Geometry: final body of the model. Coordinates: model frame, mm. A direction names the side the tool comes from. Coordinates: 2 decimals unless noted, no trailing zeros. Write each loop counter-clockwise with the first axis right and the second up, starting at its lowest first coordinate (ties: lowest second). Pieces come first, ordered by that corner, then holes. Notation, with made-up numbers: (-6.5, -10.75) - (40.5, -10.75) arc R16 ccw to (40.5, 12.25) - close; hole circle Ø2 at (36.25, -34.75). An arc over 180 degrees is marked (long way). Answer as a JSON object with one key per item and string values. Group by question number.
Item 1: Section C-C on y = 62.15. Return loops of the section in (x, z), and give its area (3 significant figures).
Item 2: Set-up query: faces 1 (the flat face through (30, 70.15, 14)), 2 (the flat face through (54, 6, 25)), 3 (the cylindrical face through (32.494, 27.794, 26.014)). Return all of +Z, -Z, +X, -X, +Y, -Y with unobstructed straight access to the full face (end or side cutting, diameter ignored); none if empty.
Item 3: First-contact query: pin 1 Ø2 at (x, y) = (34, 54) entering from -Z; pin 2 Ø2 at (x, y) = (9, 9.5) entering from +Z; pin 3 Ø3.5 at (x, y) = (8.075, 24) entering from -Z. Flat tips, straight axial feed; report the tip coordinate or a pass-through.
Item 4: Line query: line 1 along Y through (x, z) = (52.15, 24.6); line 2 along Y through (x, z) = (8, 26.2); line 3 along Y through (x, z) = (40.5, 17.75). Output: solid intervals per line, ascending. Write a range as from..to.
Item 5: Mould query, pull axis Y, two halves, no side actions, for faces 4 (the cylindrical face through (11.434, 9.081, 26.014)), 5 (the flat face through (-1.095, -1.148, 13.311)), 6 (the flat face through (59.16, 1.01, 14.37)), 7 (the flat face through (-3, 35, 13)). Classes: pulls with the +Y half, pulls with the -Y half, needs draft (parallel to the pull), parting line crosses it, or undercut.
Item 6: Section A-A on y = 24. State how many separate pieces and enclosed holes the cut face has, and give its area (3 significant figures).
Item 7: Section D-D on z = 2. Return loops of the section in (x, y), and give its area (3 significant figures).
```python
from build123d import *
from OCP.BRepFilletAPI import BRepFilletAPI_MakeChamfer

# Parameters (mm, degrees)
SKIZZE1_W                       = 60.15
SKIZZE1_H                       = 70.15
GRUNDK_RPER_DEPTH               = 24
FASE1_SIZE                      = 2
WANDUNG1_T                      = 3
SKIZZE2_R                       = 4.5
DURCHBRUCH_SERVO_DEPTH          = 101.338651576
SKIZZE4_W                       = 22
SKIZZE4_H                       = 42
SERVOFREISCHNITT_DEPTH          = 1
SCHNITT_LINEAR_AUSTRAGEN2_REACH = 102.339
SKIZZE7_R                       = 2
SKIZZE8_R                       = 3.6
SCHNITT_LINEAR_AUSTRAGEN3_DEPTH = 2
SCHNITT_LINEAR_AUSTRAGEN5_REACH = 102.339
SKIZZE3_R                       = 1.6
FASE2_SIZE                      = 5
FASE2_SIZE2                     = 0.437443318
FASE3_SIZE                      = 1
FASE3_SIZE2                     = 1.100062868


with BuildPart() as part:
    # Skizze1 → Grundkörper (new body)
    with BuildSketch(Plane.XY):
        with Locations((30.075, 35.075)):
            Rectangle(SKIZZE1_W, SKIZZE1_H)
    extrude(amount=GRUNDK_RPER_DEPTH)

    # Fase1
    fase1_edges = [part.edges().sort_by_distance(p)[0] for p in [
        (0, 70.15, 12),
        (60.15, 70.15, 12),
        (60.15, 0, 12),
        (0, 0, 12),
    ]]
    chamfer(fase1_edges, length=FASE1_SIZE)

    # Wandung1
    wandung1_openings = [part.faces().sort_by_distance(p)[0] for p in [
        (30.075, 35.075, 0),
    ]]
    offset(amount=WANDUNG1_T, openings=wandung1_openings, kind=Kind.INTERSECTION)

    # Skizze2 → Durchbruch Servo (cut, through all)
    with BuildSketch(Plane.XY.offset(27)):
        with Locations((30.075, 24)):
            Circle(SKIZZE2_R)
    extrude(amount=-DURCHBRUCH_SERVO_DEPTH, mode=Mode.SUBTRACT)

    # Skizze4 → ServoFreischnitt (cut)
    with BuildSketch(Plane(origin=(0, 0, 24), x_dir=(-1, 0, 0), z_dir=(0, 0, -1))):
        with Locations((-30.075, 35)):
            Rectangle(SKIZZE4_W, SKIZZE4_H)
    extrude(amount=-SERVOFREISCHNITT_DEPTH, mode=Mode.SUBTRACT)

    # Skizze7 → Schnitt-Linear austragen2 (cut, up to next)
    with BuildSketch(Plane.XY.offset(27), mode=Mode.PRIVATE) as schnitt_linear_austragen2_sk1:
        with Locations((8, 62.15)):
            Circle(SKIZZE7_R)
    schnitt_linear_austragen2_tool1 = extrude(schnitt_linear_austragen2_sk1.sketch, amount=-SCHNITT_LINEAR_AUSTRAGEN2_REACH, mode=Mode.PRIVATE) & part.part
    # Skizze7 → Schnitt-Linear austragen2 (cut, up to next)
    with BuildSketch(Plane.XY.offset(27), mode=Mode.PRIVATE) as schnitt_linear_austragen2_sk2:
        with Locations(Location((52.15, 62.15, 0), (0, 0, 180))):
            Circle(SKIZZE7_R)
    schnitt_linear_austragen2_tool2 = extrude(schnitt_linear_austragen2_sk2.sketch, amount=-SCHNITT_LINEAR_AUSTRAGEN2_REACH, mode=Mode.PRIVATE) & part.part
    # Skizze7 → Schnitt-Linear austragen2 (cut, up to next)
    with BuildSketch(Plane.XY.offset(27), mode=Mode.PRIVATE) as schnitt_linear_austragen2_sk3:
        with Locations((52.15, 8)):
            Circle(SKIZZE7_R)
    schnitt_linear_austragen2_tool3 = extrude(schnitt_linear_austragen2_sk3.sketch, amount=-SCHNITT_LINEAR_AUSTRAGEN2_REACH, mode=Mode.PRIVATE) & part.part
    # Skizze7 → Schnitt-Linear austragen2 (cut, up to next)
    with BuildSketch(Plane.XY.offset(27), mode=Mode.PRIVATE) as schnitt_linear_austragen2_sk4:
        with Locations(Location((8, 8, 0), (0, 0, 180))):
            Circle(SKIZZE7_R)
    schnitt_linear_austragen2_tool4 = extrude(schnitt_linear_austragen2_sk4.sketch, amount=-SCHNITT_LINEAR_AUSTRAGEN2_REACH, mode=Mode.PRIVATE) & part.part
    add(schnitt_linear_austragen2_tool1.solids().sort_by_distance((8, 62.15, 27))[0], mode=Mode.SUBTRACT)
    add(schnitt_linear_austragen2_tool2.solids().sort_by_distance((52.15, 62.15, 27))[0], mode=Mode.SUBTRACT)
    add(schnitt_linear_austragen2_tool3.solids().sort_by_distance((52.15, 8, 27))[0], mode=Mode.SUBTRACT)
    add(schnitt_linear_austragen2_tool4.solids().sort_by_distance((8, 8, 27))[0], mode=Mode.SUBTRACT)

    # Skizze8 → Schnitt-Linear austragen3 (cut)
    with BuildSketch(Plane.XY.offset(27)):
        with Locations((8, 62.15)):
            Circle(SKIZZE8_R)
        with Locations((52.15, 62.15)):
            Circle(SKIZZE8_R)
        with Locations((52.15, 8)):
            Circle(SKIZZE8_R)
        with Locations((8, 8)):
            Circle(SKIZZE8_R)
    extrude(amount=-SCHNITT_LINEAR_AUSTRAGEN3_DEPTH, mode=Mode.SUBTRACT)

    # Skizze3 → Schnitt-Linear austragen5 (cut, up to next)
    with BuildSketch(Plane.XY.offset(27), mode=Mode.PRIVATE) as schnitt_linear_austragen5_sk1:
        with Locations((8.075, 24)):
            Circle(SKIZZE3_R)
    schnitt_linear_austragen5_tool1 = extrude(schnitt_linear_austragen5_sk1.sketch, amount=-SCHNITT_LINEAR_AUSTRAGEN5_REACH, mode=Mode.PRIVATE) & part.part
    # Skizze3 → Schnitt-Linear austragen5 (cut, up to next)
    with BuildSketch(Plane.XY.offset(27), mode=Mode.PRIVATE) as schnitt_linear_austragen5_sk2:
        with Locations((52.075, 24)):
            Circle(SKIZZE3_R)
    schnitt_linear_austragen5_tool2 = extrude(schnitt_linear_austragen5_sk2.sketch, amount=-SCHNITT_LINEAR_AUSTRAGEN5_REACH, mode=Mode.PRIVATE) & part.part
    add(schnitt_linear_austragen5_tool1.solids().sort_by_distance((8.075, 24, 27))[0], mode=Mode.SUBTRACT)
    add(schnitt_linear_austragen5_tool2.solids().sort_by_distance((52.075, 24, 27))[0], mode=Mode.SUBTRACT)

    # Fase2: one chamfer whose edges measure the first distance from different faces: ONE call of the kernel's chamfer builder (chamfer() names one face for all edges)
    fase2_edges_1 = [part.edges().sort_by_distance(p)[0] for p in [
        (0, 35.075, 0),
    ]]
    fase2_side_1 = [part.faces().sort_by_distance(p)[0] for p in [
        (0, 35.075, 12),
    ]]
    fase2_edges_2 = [part.edges().sort_by_distance(p)[0] for p in [
        (30.075, 0, 0),
    ]]
    fase2_side_2 = [part.faces().sort_by_distance(p)[0] for p in [
        (30.075, 0, 12),
    ]]
    fase2_edges_3 = [part.edges().sort_by_distance(p)[0] for p in [
        (60.15, 35.075, 0),
    ]]
    fase2_side_3 = [part.faces().sort_by_distance(p)[0] for p in [
        (60.15, 35.075, 12),
    ]]
    fase2_edges_4 = [part.edges().sort_by_distance(p)[0] for p in [
        (30.075, 70.15, 0),
    ]]
    fase2_side_4 = [part.faces().sort_by_distance(p)[0] for p in [
        (30.075, 70.15, 12),
    ]]
    fase2_edges_5 = [part.edges().sort_by_distance(p)[0] for p in [
        (59.15, 1, 0),
    ]]
    fase2_side_5 = [part.faces().sort_by_distance(p)[0] for p in [
        (59.15, 1, 12),
    ]]
    fase2_edges_6 = [part.edges().sort_by_distance(p)[0] for p in [
        (1, 1, 0),
    ]]
    fase2_side_6 = [part.faces().sort_by_distance(p)[0] for p in [
        (1, 1, 12),
    ]]
    fase2_edges_7 = [part.edges().sort_by_distance(p)[0] for p in [
        (1, 69.15, 0),
    ]]
    fase2_side_7 = [part.faces().sort_by_distance(p)[0] for p in [
        (1, 69.15, 12),
    ]]
    fase2_edges_8 = [part.edges().sort_by_distance(p)[0] for p in [
        (59.15, 69.15, 0),
    ]]
    fase2_side_8 = [part.faces().sort_by_distance(p)[0] for p in [
        (59.15, 69.15, 12),
    ]]
    fase2 = BRepFilletAPI_MakeChamfer(part.part.solid().wrapped)
    for e in fase2_edges_1:
        fase2.Add(FASE2_SIZE, FASE2_SIZE2, e.wrapped, fase2_side_1[0].wrapped)  # the first distance lies on this face
    for e in fase2_edges_2:
        fase2.Add(FASE2_SIZE, FASE2_SIZE2, e.wrapped, fase2_side_2[0].wrapped)  # the first distance lies on this face
    for e in fase2_edges_3:
        fase2.Add(FASE2_SIZE, FASE2_SIZE2, e.wrapped, fase2_side_3[0].wrapped)  # the first distance lies on this face
    for e in fase2_edges_4:
        fase2.Add(FASE2_SIZE, FASE2_SIZE2, e.wrapped, fase2_side_4[0].wrapped)  # the first distance lies on this face
    for e in fase2_edges_5:
        fase2.Add(FASE2_SIZE, FASE2_SIZE2, e.wrapped, fase2_side_5[0].wrapped)  # the first distance lies on this face
    for e in fase2_edges_6:
        fase2.Add(FASE2_SIZE, FASE2_SIZE2, e.wrapped, fase2_side_6[0].wrapped)  # the first distance lies on this face
    for e in fase2_edges_7:
        fase2.Add(FASE2_SIZE, FASE2_SIZE2, e.wrapped, fase2_side_7[0].wrapped)  # the first distance lies on this face
    for e in fase2_edges_8:
        fase2.Add(FASE2_SIZE, FASE2_SIZE2, e.wrapped, fase2_side_8[0].wrapped)  # the first distance lies on this face
    add(Compound.cast(fase2.Shape()), mode=Mode.REPLACE)

    # Fase3: one chamfer whose edges measure the first distance from different faces: ONE call of the kernel's chamfer builder (chamfer() names one face for all edges)
    fase3_edges_1 = [part.edges().sort_by_distance(p)[0] for p in [
        (60.587443318, 35.075, 0),
    ]]
    fase3_side_1 = [part.faces().sort_by_distance(p)[0] for p in [
        (60.368920817, 35.075, 2.497723608),
    ]]
    fase3_edges_2 = [part.edges().sort_by_distance(p)[0] for p in [
        (59.459319136, 69.459319136, 0),
    ]]
    fase3_side_2 = [part.faces().sort_by_distance(p)[0] for p in [
        (59.307763339, 69.307763339, 2.449828985),
    ]]
    fase3_edges_3 = [part.edges().sort_by_distance(p)[0] for p in [
        (30.075, 70.587443318, 0),
    ]]
    fase3_side_3 = [part.faces().sort_by_distance(p)[0] for p in [
        (30.075, 70.368956172, 2.4973195),
    ]]
    fase3_edges_4 = [part.edges().sort_by_distance(p)[0] for p in [
        (0.690680864, 69.459319136, 0),
    ]]
    fase3_side_4 = [part.faces().sort_by_distance(p)[0] for p in [
        (0.842236661, 69.307763339, 2.449828985),
    ]]
    fase3_edges_5 = [part.edges().sort_by_distance(p)[0] for p in [
        (-0.437443318, 35.075, 0),
    ]]
    fase3_side_5 = [part.faces().sort_by_distance(p)[0] for p in [
        (-0.218920817, 35.075, 2.497723608),
    ]]
    fase3_edges_6 = [part.edges().sort_by_distance(p)[0] for p in [
        (0.690680864, 0.690680864, 0),
    ]]
    fase3_side_6 = [part.faces().sort_by_distance(p)[0] for p in [
        (0.842236661, 0.842236661, 2.449828985),
    ]]
    fase3_edges_7 = [part.edges().sort_by_distance(p)[0] for p in [
        (30.075, -0.437443318, 0),
    ]]
    fase3_side_7 = [part.faces().sort_by_distance(p)[0] for p in [
        (30.075, -0.218956172, 2.4973195),
    ]]
    fase3_edges_8 = [part.edges().sort_by_distance(p)[0] for p in [
        (59.459319136, 0.690680864, 0),
    ]]
    fase3_side_8 = [part.faces().sort_by_distance(p)[0] for p in [
        (59.307763339, 0.842236661, 2.449828985),
    ]]
    fase3 = BRepFilletAPI_MakeChamfer(part.part.solid().wrapped)
    for e in fase3_edges_1:
        fase3.Add(FASE3_SIZE, FASE3_SIZE2, e.wrapped, fase3_side_1[0].wrapped)  # the first distance lies on this face
    for e in fase3_edges_2:
        fase3.Add(FASE3_SIZE, FASE3_SIZE2, e.wrapped, fase3_side_2[0].wrapped)  # the first distance lies on this face
    for e in fase3_edges_3:
        fase3.Add(FASE3_SIZE, FASE3_SIZE2, e.wrapped, fase3_side_3[0].wrapped)  # the first distance lies on this face
    for e in fase3_edges_4:
        fase3.Add(FASE3_SIZE, FASE3_SIZE2, e.wrapped, fase3_side_4[0].wrapped)  # the first distance lies on this face
    for e in fase3_edges_5:
        fase3.Add(FASE3_SIZE, FASE3_SIZE2, e.wrapped, fase3_side_5[0].wrapped)  # the first distance lies on this face
    for e in fase3_edges_6:
        fase3.Add(FASE3_SIZE, FASE3_SIZE2, e.wrapped, fase3_side_6[0].wrapped)  # the first distance lies on this face
    for e in fase3_edges_7:
        fase3.Add(FASE3_SIZE, FASE3_SIZE2, e.wrapped, fase3_side_7[0].wrapped)  # the first distance lies on this face
    for e in fase3_edges_8:
        fase3.Add(FASE3_SIZE, FASE3_SIZE2, e.wrapped, fase3_side_8[0].wrapped)  # the first distance lies on this face
    add(Compound.cast(fase3.Shape()), mode=Mode.REPLACE)


solid = part.part
```
Checks:
{
 "1": {"outline": "(-3, 0) - (-1.54, 0) - (-0.35, 1) - (0, 5) - (0, 24) - (6, 24) - (6, 25) - (4.4, 25) - (4.4, 27) - (-3, 27) - close; (10, 24) - (50.15, 24) - (50.15, 25) - (48.55, 25) - (48.55, 27) - (11.6, 27) - (11.6, 25) - (10, 25) - close; (54.15, 24) - (60.15, 24) - (60.15, 5) - (60.5, 1) - (61.69, 0) - (63.15, 0) - (63.15, 27) - (55.75, 27) - (55.75, 25) - (54.15, 25) - close", "area": "302 mm^2"},
 "2": {"face 1": "-Z", "face 2": "+Z", "face 3": "+Z, -Z"},
 "3": {"pin 1": "z = 25", "pin 2": "z = 25", "pin 3": "z = 24"},
 "4": {"line 1": "-3..6, 10..22.4, 25.6..60.15, 64.15..73.15", "line 2": "-3..4.4, 11.6..22.4, 25.6..58.55, 65.75..73.15", "line 3": "-3..0, 70.15..73.15"},
 "5": {"face 4": "undercut", "face 5": "pulls with the -Y half", "face 6": "undercut", "face 7": "needs draft"},
 "6": {"separate pieces": "4", "enclosed holes": "0", "area": "280 mm^2"},
 "7": {"outline": "(-3, 0.76) - (0.76, -3) - (59.39, -3) - (63.15, 0.76) - (63.15, 69.39) - (59.39, 73.15) - (0.76, 73.15) - (-3, 69.39) - close; hole (-0.26, 1.89) - (1.89, -0.26) - (58.26, -0.26) - (60.41, 1.89) - (60.41, 68.26) - (58.26, 70.41) - (1.89, 70.41) - (-0.26, 68.26) - close", "area": "730 mm^2"}
}
